The figure shows three views and two pictorial views of one solid part (mm, origin at its lowest corner). Answer the questions. A direction names the side the tool comes from. Give positions to 0.01 mm unless a question says otherwise; leave off trailing zeros. Write each loop counter-clockwise with the first axis right and the second up, starting at its lowest first coordinate (ties: lowest second). Pieces come first, ordered by that corner, then holes. Notation, with made-up numbers: (66.25, 75) - (81.25, 75) arc R22 cw to (81.25, 112) - close; hole circle Ø7 at (71, 59). An arc over 180 degrees is marked (long way). One line per question, with ' | ' between items. Start each with the question number.
1. A cutting plane is placed at D-D (z = 151). Determine the outline of the cut face in (x, y), then the cut area to 3 significant figures.
2. Given P1, Ø5, axis at x = 109.5, y = 132, coming from the -Z side; P2, Ø6, axis at y = 126.5, z = 176.5, coming from the +X side; P3, Ø10, axis at x = 48.5, y = 113, coming from the +Z side, each flat-ended and moving along its own axis, determine where each tip first touches the part or whether it passes through.
3. For the marked faces 1 and 2, determine the directions among +Z, -Z, +X, -X, +Y, -Y from which every point of the face is accessible in a straight line to the end or side of a thin tool.
4. Find the intervals of material crossed by L1, parallel to X at y = 270, z = 100; L2, parallel to Y at x = 188.5, z = 71.5, in increasing order. Write a range as from..to.
5. A cutting plane is placed at B-B (x = 100). Determine the outline of the cut face in (y, z), then the cut area to 4 significant figures.
6. A cutting plane is placed at A-A (z = 100). Determine the outline of the cut face in (x, y).
7. A cutting plane is placed at C-C (y = 125). Determine the outline of the cut face in (x, z).
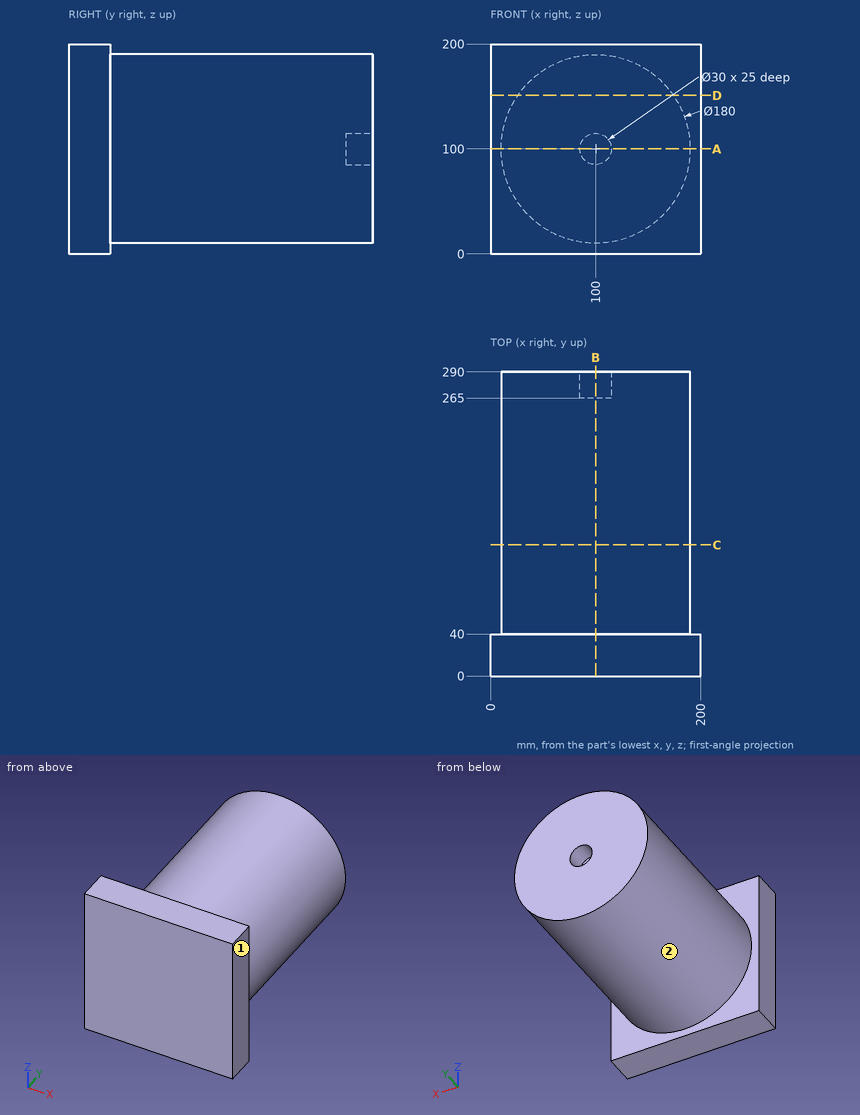
Determined:
1) outline: (0, 0) - (200, 0) - (200, 40) - (174.16, 40) - (174.16, 290) - (25.84, 290) - (25.84, 40) - (0, 40) - close | area: 45,100 mm2
2) P1: z = 10.27 | P2: x = 151.94 | P3: z = 177.06
3) face 1: +Z, -Z, +X, +Y, -Y | face 2: +Y
4) L1: 10..85, 115..190 | L2: 0..40
5) outline: (0, 0) - (40, 0) - (40, 10) - (290, 10) - (290, 85) - (265, 85) - (265, 115) - (290, 115) - (290, 190) - (40, 190) - (40, 200) - (0, 200) - close | area: 52,250 mm2
6) outline: (0, 0) - (200, 0) - (200, 40) - (190, 40) - (190, 290) - (115, 290) - (115, 265) - (85, 265) - (85, 290) - (10, 290) - (10, 40) - (0, 40) - close
7) outline: circle Ø180 at (100, 100)
